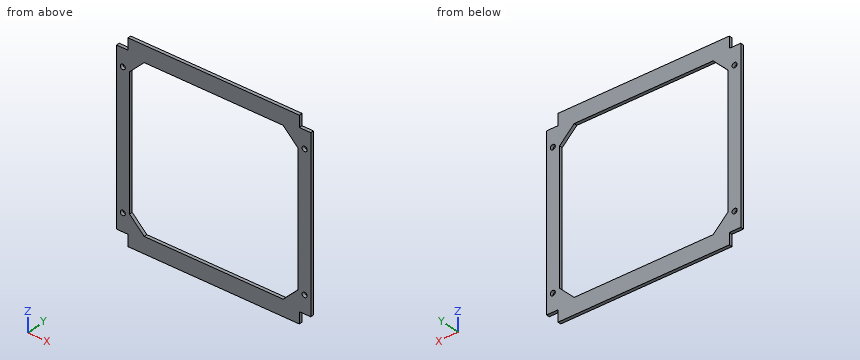
from build123d import *

# Parameters (mm, degrees)
BOSS_EXTRUDE1_DEPTH      = 1.56
CUT_EXTRUDE1_DEPTH       = 1.56
M2_CLEARANCE_HOLE1_D     = 2.4
M2_CLEARANCE_HOLE1_DEPTH = 38.1
M2_CLEARANCE_HOLE1_TIP   = 0.721032743


with BuildPart() as part:
    # Sketch1 → Boss-Extrude1 (new body)
    with BuildSketch(Plane(origin=(0, 0, 0), x_dir=(1, 0, 0), z_dir=(0, 1, 0))):
        Polygon((-41, -41), (-46.5, -41), (-46.5, 41), (-41, 41), (-41, 46.5), (41, 46.5), (41, 41), (46.5, 41), (46.5, -41), (41, -41), (41, -46.5), (-41, -46.5), align=None)
    extrude(amount=BOSS_EXTRUDE1_DEPTH)

    # Sketch2 → Cut-Extrude1 (cut)
    with BuildSketch(Plane(origin=(0, 1.56, 0), x_dir=(1, 0, 0), z_dir=(0, 1, 0))):
        Polygon((-40.243314804, 31.704788024), (-33.243314804, 38.704788024), (33.243314804, 38.704788024), (40.243314804, 31.704788024), (40.243314804, -31.704788024), (33.243314804, -38.704788024), (-33.243314804, -38.704788024), (-40.243314804, -31.704788024), align=None)
    extrude(amount=-CUT_EXTRUDE1_DEPTH, mode=Mode.SUBTRACT)

    # M2 Clearance Hole1
    with Locations(Plane(origin=(0, 1.56, 0), x_dir=(1, 0, 0), z_dir=(0, 1, 0))):
        with Locations((-43.5, -32.5), (-43.5, 32.5), (43.5, 32.5), (43.5, -32.5)):
            Hole(M2_CLEARANCE_HOLE1_D / 2, depth=M2_CLEARANCE_HOLE1_DEPTH)
            with Locations((0, 0, -(M2_CLEARANCE_HOLE1_DEPTH + M2_CLEARANCE_HOLE1_TIP / 2))):  # 118° drill point
                Cone(0, M2_CLEARANCE_HOLE1_D / 2, M2_CLEARANCE_HOLE1_TIP, mode=Mode.SUBTRACT)


solid = part.part
Design review of the part built by this model. Coordinates are the model's own, in mm. Round coordinates to 2 decimals unless told otherwise and drop trailing zeros. Order: outer loops, then holes, each group sorted by start corner. A loop starts at its lowest first (then second) coordinate and runs counter-clockwise, first axis right, second up. Notation, with made-up numbers: M 55.25,5.5 L 85.25,5.5 A36 ccw 85.25,44.5 Z; hole C 87,-4 d2. An arc over 180 degrees is marked long. Answer as CSV lines item,"result". Start each with the question number.
1) Add section B-B (z = -5.5). Give the boundary of the cut face in (x, y), then the cut area to 3 significant figures.
2) Add section C-C (y = 0.25). Give the boundary of the cut face in (x, z).
3) Add section D-D (x = 43.5). Give the boundary of the cut face in (y, z).
4) Wall thickness on line 1 along Z through (x, y) = (43.5, 0.7); line 2 along X through (y, z) = (1.35, -10.5); line 3 along Z through (x, y) = (30, 0.6): over which ranges is each line inside the solid? List them lowest first. Write a range as [from, to].
5) For pin 1 Ø0.8 at (x, y) = (42.5, 0.5) entering from +Z; pin 2 Ø0.5 at (y, z) = (0.5, 43) entering from +X; pin 3 Ø0.8 at (y, z) = (0.5, 42.5) entering from -X, all flat-tipped, find the tip position at first contact; note any pin that passes through.
6) Add section A-A (x = -25). Give the boundary of the cut face in (y, z), then the cut area to 3 significant figures.
Resolved:
1,outline,"M -46.5,0 L -40.24,0 L -40.24,1.56 L -46.5,1.56 Z; M 40.24,0 L 46.5,0 L 46.5,1.56 L 40.24,1.56 Z"
1,area,"19.5 mm^2"
2,outline,"M -46.5,-41 L -41,-41 L -41,-46.5 L 41,-46.5 L 41,-41 L 46.5,-41 L 46.5,41 L 41,41 L 41,46.5 L -41,46.5 L -41,41 L -46.5,41 Z; hole C -43.5,-32.5 d2.4; hole C -43.5,32.5 d2.4; hole M -40.24,-31.7 L -33.24,-38.7 L 33.24,-38.7 L 40.24,-31.7 L 40.24,31.7 L 33.24,38.7 L -33.24,38.7 L -40.24,31.7 Z; hole C 43.5,-32.5 d2.4; hole C 43.5,32.5 d2.4"
3,outline,"M 0,-41 L 1.56,-41 L 1.56,-33.7 L 0,-33.7 Z; M 0,-31.3 L 1.56,-31.3 L 1.56,31.3 L 0,31.3 Z; M 0,33.7 L 1.56,33.7 L 1.56,41 L 0,41 Z"
4,line 1,"[-41, -33.7], [-31.3, 31.3], [33.7, 41]"
4,line 2,"[-46.5, -40.24], [40.24, 46.5]"
4,line 3,"[-46.5, -38.7], [38.7, 46.5]"
5,pin 1,"z = 41"
5,pin 2,"x = 41"
5,pin 3,"x = -41"
6,outline,"M 0,-46.5 L 1.56,-46.5 L 1.56,-38.7 L 0,-38.7 Z; M 0,38.7 L 1.56,38.7 L 1.56,46.5 L 0,46.5 Z"
6,area,"24.3 mm^2"
